Could you check a few things on this drawing? It's one solid part, dimensions in mm from its lowest x, y, z. A direction names the side the tool comes from. Give positions to 0.01 mm unless a question says otherwise; leave off trailing zeros. Write each loop counter-clockwise with the first axis right and the second up, starting at its lowest first coordinate (ties: lowest second). Pieces come first, ordered by that corner, then holes. Notation, with made-up numbers: (32, 76.25) - (81, 76.25) arc R9 ccw to (81, 92.25) - close; hole circle Ø11 at (58.5, 45.5). An arc over 180 degrees is marked (long way). One line per item, written item: value. Start each with the question number.
1) Imagine slicing it at B-B on y = 30. Write out the boundary of the cut face in (x, z).
2) We'd pull the mould along X, two halves only. Please class the marked faces 1, 2 and 3: +X half, -X half, draft (parallel to the pull), parting line (faces both ways), or undercut.
3) Imagine slicing it at C-C on x = 15.5. Write out the boundary of the cut face in (y, z).
4) Imagine slicing it at D-D on z = 9.5. Write out the boundary of the cut face in (x, y).
5) On a 3-axis mill with a long thin cutter (end or side, diameter ignored), from which of +Z, -Z, +X, -X, +Y, -Y can I reach the whole of each face in a straight line? I mean the marked faces 4 and 5. Say none if no direction works.
6) I'm going to push a flat-ended pin straight in: P1, Ø12, axis at x = 33.5, y = 19, coming from the +Z side. Where does the tip first touch, or does it pass through?
7) Imagine slicing it at A-A on x = 42.5. Write out the boundary of the cut face in (y, z), plus the area to 3 significant figures.
8) Please list where these lines run through material, in increasing order: L1, parallel to Y at x = 18.5, z = 7; L2, parallel to Y at x = 48, z = 8.5; L3, parallel to X at y = 20, z = 7.25. Write a range as [from, to].
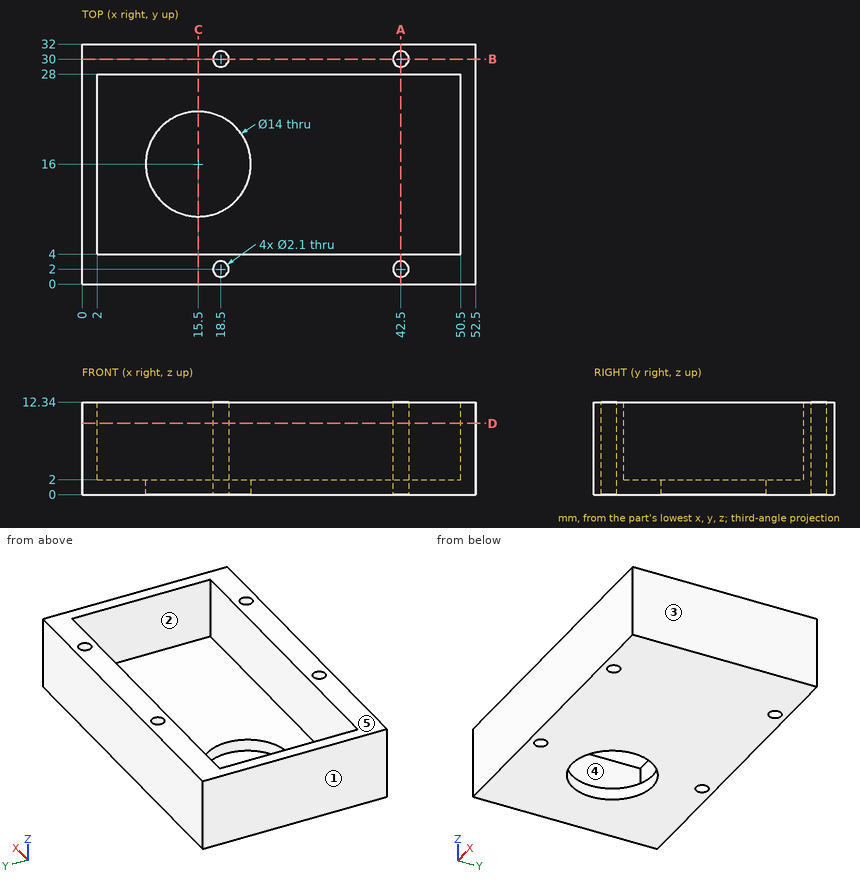
Numbers:
1. outline: (0, 0) - (17.45, 0) - (17.45, 12.34) - (0, 12.34) - close; (19.55, 0) - (41.45, 0) - (41.45, 12.34) - (19.55, 12.34) - close; (43.55, 0) - (52.5, 0) - (52.5, 12.34) - (43.55, 12.34) - close
2. face 1: -X half
2. face 2: undercut
2. face 3: +X half
3. outline: (0, 0) - (9, 0) - (9, 2) - (4, 2) - (4, 12.34) - (0, 12.34) - close; (23, 0) - (32, 0) - (32, 12.34) - (28, 12.34) - (28, 2) - (23, 2) - close
4. outline: (0, 0) - (52.5, 0) - (52.5, 32) - (0, 32) - close; hole (2, 4) - (50.5, 4) - (50.5, 28) - (2, 28) - close; hole circle Ø2.1 at (18.5, 2); hole circle Ø2.1 at (18.5, 30); hole circle Ø2.1 at (42.5, 2); hole circle Ø2.1 at (42.5, 30)
5. face 4: +Z
5. face 5: +Z, +X, -X, +Y, -Y
6. P1: z = 2
7. outline: (0, 0) - (0.95, 0) - (0.95, 12.34) - (0, 12.34) - close; (3.05, 0) - (28.95, 0) - (28.95, 12.34) - (28, 12.34) - (28, 2) - (4, 2) - (4, 12.34) - (3.05, 12.34) - close; (31.05, 0) - (32, 0) - (32, 12.34) - (31.05, 12.34) - close
7. area: 94.9 mm^2
8. L1: [0, 0.95], [3.05, 4], [28, 28.95], [31.05, 32]
8. L2: [0, 4], [28, 32]
8. L3: [0, 2], [50.5, 52.5]
